Can you work these out from the model? Positions are in its coordinate system, mm. Coordinates: 2 decimals unless noted, no trailing zeros. Loops run counter-clockwise (first coordinate to the right, second up) from the corner with the lowest first, then second, coordinate; pieces in that order, holes last.
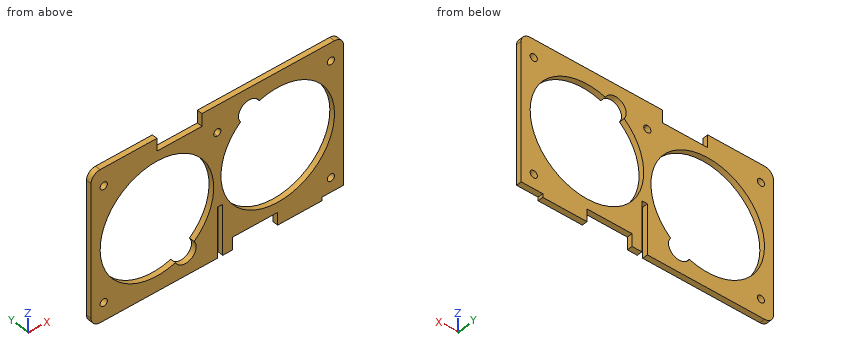
```python
from build123d import *

# Parameters (mm, degrees)
F0_R     = 2
F1_DEPTH = 3


with BuildPart() as f1:
    # F0 (on Front) → F1 (new body)
    with BuildSketch(Plane.XZ):
        with BuildLine():
            ThreePointArc((-70, -37), (-68.535534, -40.535534), (-65, -42))
            Line((-65, -42), (0, -42))
            Line((0, -42), (0, -14))
            Line((0, -14), (0, 25))
            ThreePointArc((0, 25), (-2, 27), (0, 29))
            Line((0, 29), (0, 42))
            Line((0, 42), (-8.5, 42))
            Line((-8.5, 42), (-8.5, 35))
            Line((-8.5, 35), (-33.5, 35))
            Line((-33.5, 35), (-33.5, 42))
            Line((-33.5, 42), (-65, 42))
            ThreePointArc((-65, 42), (-68.535534, 40.535534), (-70, 37))
            Line((-70, 37), (-70, -37))
        make_face()
        with Locations((-63, -32)):
            Circle(F0_R, mode=Mode.SUBTRACT)
        with BuildLine():
            ThreePointArc((-23.208248, -31.771292), (-49.25, 25.2798), (-12.863181, -25.798565))
            ThreePointArc((-12.863181, -25.798565), (-14.75, -34.475953), (-23.208248, -31.771292))
        make_face(mode=Mode.SUBTRACT)
        with Locations((-63, 32)):
            Circle(F0_R, mode=Mode.SUBTRACT)
        with BuildLine():
            Line((0, 25), (0, -14))
            Line((0, -14), (3, -14))
            Line((3, -14), (3, -42))
            Line((3, -42), (8.5, -42))
            Line((8.5, -42), (8.5, -35))
            Line((8.5, -35), (33.5, -35))
            Line((33.5, -35), (33.5, -42))
            Line((33.5, -42), (58, -42))
            Line((58, -42), (58, -40))
            Line((58, -40), (70, -40))
            Line((70, -40), (70, 37))
            ThreePointArc((70, 37), (68.535534, 40.535534), (65, 42))
            Line((65, 42), (0, 42))
            Line((0, 42), (0, 29))
            ThreePointArc((0, 29), (1.414214, 28.414214), (2, 27))
            ThreePointArc((2, 27), (1.414214, 25.585786), (0, 25))
        make_face()
        with Locations((63, -32)):
            Circle(F0_R, mode=Mode.SUBTRACT)
        with BuildLine():
            ThreePointArc((23.208248, 31.771292), (49.25, -25.2798), (12.863181, 25.798565))
            ThreePointArc((12.863181, 25.798565), (14.75, 34.475953), (23.208248, 31.771292))
        make_face(mode=Mode.SUBTRACT)
        with Locations((63, 32)):
            Circle(F0_R, mode=Mode.SUBTRACT)
    extrude(amount=F1_DEPTH)


solid = f1.part
```
Item 1: Suppose I cut it at B-B, the plane y = -2.5. Count the separate pieces of the cut face and the enclosed holes in it, plus the area to 3 significant figures.
Results are:
separate pieces: 1
enclosed holes: 7
area: 4,870 mm2
Item 2: I need wall thicknesses on line 1 along X through (y, z) = (-0.6, -5); line 2 along X through (y, z) = (-2.2, 9); line 3 along X through (y, z) = (-1.05, 26.5). Which ranges of each line are inside material? Lowest first, please.
Results are:
line 1: x = -70 to -64.86, -2.14 to 2.79, 64.21 to 70
line 2: x = -70 to -63.02, -3.98 to 2.79, 64.21 to 70
line 3: x = -70 to -46.92, -20.08 to -1.94, 1.94 to 12.43, 53.3 to 70
Item 3: I'm going to push flat-ended pins straight in: P1, Ø3.5, axis at x = -63, z = -32, coming from the +Y side; P2, Ø1.5, axis at x = -18.5, y = -2, coming from the +Z side; P3, Ø1.5, axis at y = -1, z = -39.5, coming from the -X side; P4, Ø1.5, axis at y = -2, z = 38.5, coming from the +X side. Where does each tip first touch, or does it pass through?
Results are:
P1: passes through
P2: stops at z = 35
P3: stops at x = -69.68
P4: stops at x = 69.94
Item 4: Suppose I cut it at C-C, the plane x = 17.75. Please give me the cut outline in (y, z), plus the area to 3 significant figures.
Results are:
outline: (-3, -35) - (0, -35) - (0, -25.28) - (-3, -25.28) - close; (-3, 35.28) - (0, 35.28) - (0, 42) - (-3, 42) - close
area: 49.3 mm2
Item 5: Suppose I cut it at A-A, the plane z = -0.5. Please give me the cut outline in (x, y).
Results are:
outline: (-70, -3) - (-64.96, -3) - (-64.96, 0) - (-70, 0) - close; (-2.04, -3) - (2.1, -3) - (2.1, 0) - (-2.04, 0) - close; (64.9, -3) - (70, -3) - (70, 0) - (64.9, 0) - close
Item 6: Suppose I cut it at D-D, the plane x = -47. Please give me the cut outline in (y, z).
Results are:
outline: (-3, -42) - (0, -42) - (0, -30.46) - (-3, -30.46) - close; (-3, 26.46) - (0, 26.46) - (0, 42) - (-3, 42) - close
